from build123d import *

# Parameters (mm, degrees)
EXTRUDE1_DEPTH = 177.8
EXTRUDE2_DEPTH = 387.35


with BuildPart() as part:
    # Sketch1 → Extrude1 (new, symmetric)
    with BuildSketch(Plane.XY):
        with BuildLine():
            Line((0, 0), (0, 25.4))
            Line((0, 25.4), (1.5875, 25.4))
            Line((1.5875, 25.4), (1.5875, 1.5875))
            ThreePointArc((1.5875, 1.5875), (13.671867582, 0.546246178), (25.4, -2.546820159))
            Line((25.4, -2.546820159), (25.4, -4.781862636))
            ThreePointArc((25.4, -4.781862636), (12.923101507, -1.205874633), (0, 0))
        make_face()
    extrude(amount=EXTRUDE1_DEPTH, both=True)

    # Sketch2 → Extrude2 (cut)
    with BuildSketch(Plane.ZY):
        Polygon((177.8, 25.4), (153.9875, 25.4), (177.8, 1.5875), align=None)
    extrude2 = extrude(amount=-EXTRUDE2_DEPTH, mode=Mode.SUBTRACT)

    # Mirror2: Extrude2 across plane
    add(extrude2.mirror(Plane(origin=(0, 0, 0), x_dir=(1, 0, 0), z_dir=(0, 0, -1))), mode=Mode.SUBTRACT)


solid = part.part
Verification items for the finished model (mm, model axes). A direction names the side the tool comes from. Round coordinates to 2 decimals unless told otherwise and drop trailing zeros. Loops run counter-clockwise (first coordinate to the right, second up) from the corner with the lowest first, then second, coordinate; pieces in that order, holes last. Notation, with made-up numbers: (89.25, -18.5) - (130.25, -18.5) arc R25 ccw to (130.25, 5.5) - close; hole circle Ø4 at (-15, 84). An arc over 180 degrees is marked (long way). Answer in a Markdown table with one row per item. Add a question column.
Q1. Section check B-B on x = 7.5. Enter the section's corners in (y, z).
Q2. Tool access check on faces 1 (the face through (14, -1, 177.8)), 2 (the face through (1.588, 14, 2)). Record the directions out of +Z, -Z, +X, -X, +Y, -Y that give a thin tool (end or side, any length) a straight path to the whole face; none if there is none.
Q3. Section check A-A on z = 46.5. Enter the section's corners in (x, y).
Q4. Material ranges on line 1 (Y direction, x = 2, z = 151.5); line 2 (X direction, y = 22.5, z = -66); line 3 (Y direction, x = 23, z = -26), recorded low to high.
Q5. Section check C-C on y = 22.5. Enter the section's corners in (x, z).
Q6. Gauge pin test, flat ends, axial feed: pin 1 (12 mm diameter, centred on x = 10, y = 3.5, fed in from -Z); pin 2 (12 mm diameter, centred on y = 18, z = -76.5, fed in from +X); pin 3 (10 mm diameter, centred on x = 12, z = -91, fed in from -Y). Record the tip position at first contact, or that the pin passes through.
Found:
| question | item | result |
|---|---|---|
| 1 | outline | (-0.4, -177.8) - (1.34, -177.8) - (1.34, 177.8) - (-0.4, 177.8) - close |
| 2 | face 1 | +Z, +X, -X, +Y, -Y |
| 2 | face 2 | +Z, -Z, +X, +Y |
| 3 | outline | (0, 0) arc R69.85 cw to (25.4, -4.78) - (25.4, -2.55) arc R70.64 ccw to (1.59, 1.59) - (1.59, 25.4) - (0, 25.4) - close |
| 4 | line 1 | y = -0.03 to 1.59 |
| 4 | line 2 | x = 0 to 1.59 |
| 4 | line 3 | y = -3.9 to -1.74 |
| 5 | outline | (0, -156.89) - (1.59, -156.89) - (1.59, 156.89) - (0, 156.89) - close |
| 6 | pin 1 | stops at z = -177.8 |
| 6 | pin 2 | stops at x = 1.59 |
| 6 | pin 3 | stops at y = -2.1 |
